Input: dimensioned drawing with shaded views. Units: mm. Origin: part minimum x, y, z. A direction names the side the tool comes from. Give positions to 0.01 mm unless a question says otherwise; leave off trailing zeros. Loops run counter-clockwise (first coordinate to the right, second up) from the corner with the lowest first, then second, coordinate; pieces in that order, holes last.
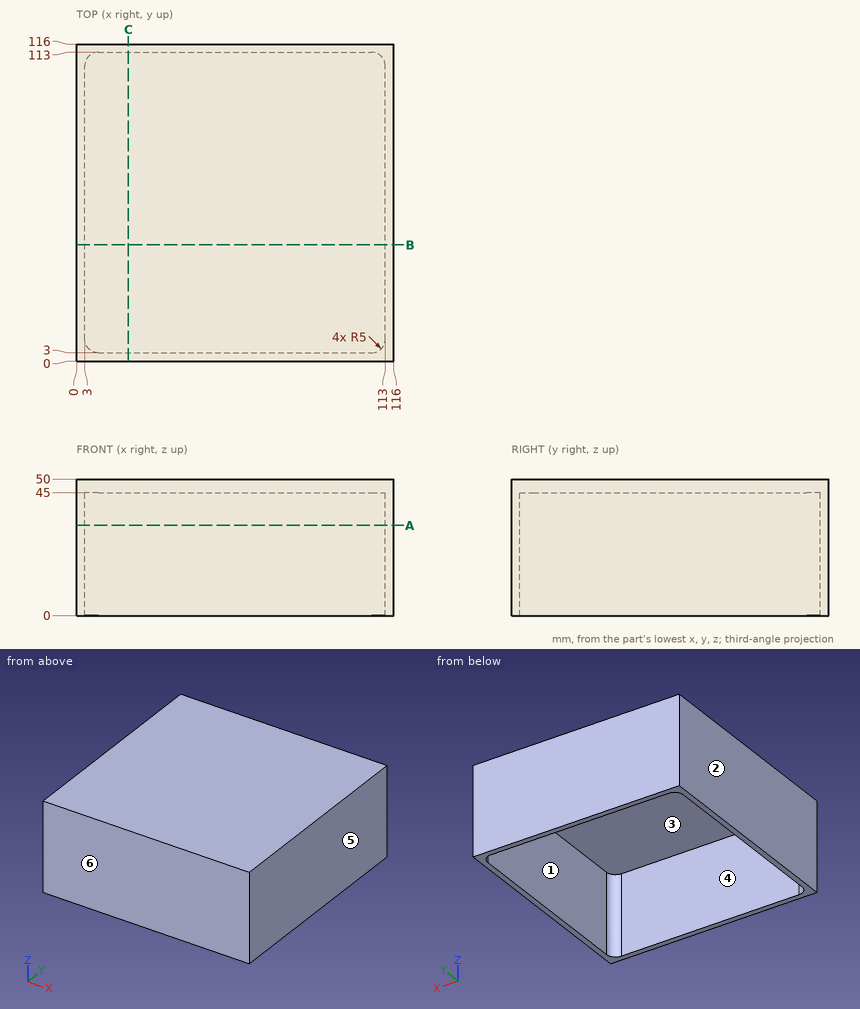
(1) Reachability of the marked faces 1 and 2 from +Z, -Z, +X, -X, +Y, -Y: full face, straight path, thin tool, end or side. Return the list, or none.
A:
face 1: -Z
face 2: +Z, -Z, -X, +Y, -Y
(2) Section A-A, the plane z = 33. Return the cut outline in (x, y).
A:
outline: (0, 0) - (116, 0) - (116, 116) - (0, 116) - close; hole (3, 8) arc R5 ccw to (8, 3) - (108, 3) arc R5 ccw to (113, 8) - (113, 108) arc R5 ccw to (108, 113) - (8, 113) arc R5 ccw to (3, 108) - close
(3) Mould query, pull axis X, two halves, no side actions, for the marked faces 3, 4, 5 and 6. Classes: pulls with the +X half, pulls with the -X half, needs draft (parallel to the pull), parting line crosses it, or undercut.
A:
face 3: undercut
face 4: undercut
face 5: pulls with the +X half
face 6: needs draft
(4) First-contact query: pin 1 (1 mm diameter, centred on x = 99.5, y = 41.5, fed in from -Z). Flat tip, straight axial feed; report the tip coordinate or a pass-through.
A:
pin 1: stops at z = 45
(5) Section B-B, the plane y = 42.5. Return the cut outline in (x, z), then the cut area to 3 significant figures.
A:
outline: (0, 0) - (3, 0) - (3, 45) - (113, 45) - (113, 0) - (116, 0) - (116, 50) - (0, 50) - close
area: 850 mm2
(6) Ray query, line 1 along Y through (x, z) = (51.5, 23); line 2 along Z through (x, y) = (33, 53). Return the intervals inside material, ascending.
A:
line 1: y = 0 to 3, 113 to 116
line 2: z = 45 to 50
